```python
from build123d import *

# Parameters (mm, degrees)
SKETCH_1_W               = 100
SKETCH_1_H               = 228
EXTRUDE_1_DEPTH          = 1
SKETCH_2_W               = 96
SKETCH_2_H               = 1
SKETCH_2_W_2             = 1
SKETCH_2_H_2             = 224
EXTRUDE_2_DEPTH          = 23
FILLET_1_R               = 0.9
FILLET_2_R               = 1.9
CUT_EXTRUDE_1_DEPTH      = 22
CUT_EXTRUDE_1_DEPTH_BACK = 22
FILLET_3_R               = 1
SKETCH_4_R               = 5
CUT_EXTRUDE_2_DEPTH      = 10
SKETCH_5_R               = 2
CUT_EXTRUDE_3_DEPTH      = 30
SKETCH_6_R               = 2
CUT_EXTRUDE_4_DEPTH      = 30
SKETCH_7_R               = 2
CUT_EXTRUDE_5_DEPTH      = 30
SKETCH_8_R               = 2
CUT_EXTRUDE_6_DEPTH      = 30
CUT_EXTRUDE_7_DEPTH      = 10


with BuildPart() as part:
    # Эскиз1 → Бобышка-Вытянуть1 (new body)
    with BuildSketch(Plane.XY):
        with Locations((50, 114)):
            Rectangle(SKETCH_1_W, SKETCH_1_H)
    extrude(amount=EXTRUDE_1_DEPTH)

    # Эскиз2 → Бобышка-Вытянуть2 (add)
    with BuildSketch(Plane.XY.offset(1)):
        with Locations((50, 227.5)):
            Rectangle(SKETCH_2_W, SKETCH_2_H)
        with Locations((50, 0.5)):
            Rectangle(SKETCH_2_W, SKETCH_2_H)
        with Locations((99.5, 114)):
            Rectangle(SKETCH_2_W_2, SKETCH_2_H_2)
        with Locations((0.5, 114)):
            Rectangle(SKETCH_2_W_2, SKETCH_2_H_2)
    extrude(amount=EXTRUDE_2_DEPTH)

    # Скругление1
    fillet_1_edges = [part.edges().sort_by_distance(p)[0] for p in [
        (50, 227, 1),
        (50, 1, 1),
        (99, 114, 1),
        (1, 114, 1),
    ]]
    fillet(fillet_1_edges, radius=FILLET_1_R)

    # Скругление2
    # the kernel refuses this fillet: 1.9 mm, written as the material it takes off along each edge
    with BuildSketch(Plane(origin=(-4.75, 228, 0), x_dir=(0, -1, 0), z_dir=(1, 0, 0)), Plane(origin=(104.75, 0, 0), x_dir=(0, 1, 0), z_dir=(-1, 0, 0))) as fillet_2_piece_1:
        with BuildLine():
            CenterArc((FILLET_2_R, -FILLET_2_R), FILLET_2_R, 90, 90)
            Line((0, -FILLET_2_R), (0, 0))
            Line((0, 0), (FILLET_2_R, 0))
        make_face()
    extrude(amount=109.5, mode=Mode.SUBTRACT)
    with BuildSketch(Plane(origin=(100, 232.75, 0), x_dir=(-1, 0, 0), z_dir=(0, -1, 0))) as fillet_2_piece_2:
        with BuildLine():
            CenterArc((FILLET_2_R, -FILLET_2_R), FILLET_2_R, 90, 90)
            Line((0, -FILLET_2_R), (0, 0))
            Line((0, 0), (FILLET_2_R, 0))
        make_face()
    extrude(amount=237.5, mode=Mode.SUBTRACT)
    with BuildSketch(Plane(origin=(0, -4.75, 0), x_dir=(0, 0, 1), z_dir=(0, 1, 0))) as fillet_2_piece_3:
        with BuildLine():
            CenterArc((FILLET_2_R, FILLET_2_R), FILLET_2_R, 180, 90)
            Line((0, FILLET_2_R), (0, 0))
            Line((0, 0), (FILLET_2_R, 0))
        make_face()
    extrude(amount=237.5, mode=Mode.SUBTRACT)

    # Эскиз3 → Вырез-Вытянуть1 (cut, two sides: drawn at the far end of the back side and taken through both)
    with BuildSketch(Plane.XY.offset(1).offset(-CUT_EXTRUDE_1_DEPTH_BACK)):
        with BuildLine():
            Line((0.226679947, 226), (0.226679947, 227.773320053))
            Line((0.226679947, 227.773320053), (2, 227.773320053))
            Line((2, 227.773320053), (2, 226.329128785))
            ThreePointArc((2, 226.329128785), (2.076776695, 225.923223305), (1.670871215, 226))
            Line((1.670871215, 226), (0.226679947, 226))
        make_face()
        with BuildLine():
            Line((118, 226.329128785), (118, 227.773320053))
            Line((118, 227.773320053), (119.773320053, 227.773320053))
            Line((119.773320053, 227.773320053), (119.773320053, 226))
            Line((119.773320053, 226), (118.329128785, 226))
            ThreePointArc((118.329128785, 226), (117.923223305, 225.923223305), (118, 226.329128785))
        make_face()
        with BuildLine():
            Line((2, 1.670871215), (2, 0.226679947))
            Line((2, 0.226679947), (0.226679947, 0.226679947))
            Line((0.226679947, 0.226679947), (0.226679947, 2))
            Line((0.226679947, 2), (1.670871215, 2))
            ThreePointArc((1.670871215, 2), (2.076776695, 2.076776695), (2, 1.670871215))
        make_face()
        with BuildLine():
            Line((119.773320053, 2), (119.773320053, 0.226679947))
            Line((119.773320053, 0.226679947), (118, 0.226679947))
            Line((118, 0.226679947), (118, 1.670871215))
            ThreePointArc((118, 1.670871215), (117.923223305, 2.076776695), (118.329128785, 2))
            Line((118.329128785, 2), (119.773320053, 2))
        make_face()
    extrude(amount=CUT_EXTRUDE_1_DEPTH + CUT_EXTRUDE_1_DEPTH_BACK, mode=Mode.SUBTRACT)

    # Скругление3
    fillet_3_edges = [part.edges().sort_by_distance(p)[0] for p in [
        (98, 227.5, 24),
        (2, 227.5, 24),
        (98, 0.5, 24),
        (2, 0.5, 24),
        (99.5, 2, 24),
        (99.5, 226, 24),
        (0.5, 226, 24),
        (0.5, 2, 24),
    ]]
    fillet(fillet_3_edges, radius=FILLET_3_R)

    # Эскиз4 → Вырез-Вытянуть2 (cut)
    with BuildSketch(Plane.XY.offset(1)):
        with Locations((33.703708686, 202)):
            Circle(SKETCH_4_R)
        with Locations((33.703708686, 177)):
            Circle(SKETCH_4_R)
        with Locations((33.703708686, 152)):
            Circle(SKETCH_4_R)
        with Locations((33.703708686, 127)):
            Circle(SKETCH_4_R)
        with Locations((33.703708686, 102)):
            Circle(SKETCH_4_R)
        with Locations((33.703708686, 77)):
            Circle(SKETCH_4_R)
        with Locations((33.703708686, 52)):
            Circle(SKETCH_4_R)
        with Locations((33.703708686, 27)):
            Circle(SKETCH_4_R)
        with Locations((57.851854343, 20.529523872)):
            Circle(SKETCH_4_R)
        with Locations((57.851854343, 45.529523872)):
            Circle(SKETCH_4_R)
        with Locations((57.851854343, 70.529523872)):
            Circle(SKETCH_4_R)
        with Locations((57.851854343, 95.529523872)):
            Circle(SKETCH_4_R)
        with Locations((57.851854343, 120.529523872)):
            Circle(SKETCH_4_R)
        with Locations((57.851854343, 145.529523872)):
            Circle(SKETCH_4_R)
        with Locations((57.851854343, 170.529523872)):
            Circle(SKETCH_4_R)
        with Locations((57.851854343, 195.529523872)):
            Circle(SKETCH_4_R)
        with Locations((82, 202)):
            Circle(SKETCH_4_R)
        with Locations((82, 177)):
            Circle(SKETCH_4_R)
        with Locations((82, 152)):
            Circle(SKETCH_4_R)
        with Locations((82, 127)):
            Circle(SKETCH_4_R)
        with Locations((82, 102)):
            Circle(SKETCH_4_R)
        with Locations((82, 77)):
            Circle(SKETCH_4_R)
        with Locations((82, 52)):
            Circle(SKETCH_4_R)
        with Locations((82, 27)):
            Circle(SKETCH_4_R)
    extrude(amount=-CUT_EXTRUDE_2_DEPTH, mode=Mode.SUBTRACT)

    # Эскиз5 → Вырез-Вытянуть3 (cut)
    with BuildSketch(Plane(origin=(0, 228, 0), x_dir=(1, 0, 0), z_dir=(0, 1, 0))):
        with Locations(Location((16, -12, 0), (0, 0, 270))):
            Circle(SKETCH_5_R)
        with Locations(Location((84, -12, 0), (0, 0, 270))):
            Circle(SKETCH_5_R)
        with Locations((84, 252)):
            Circle(SKETCH_5_R)
        with Locations((16, 252)):
            Circle(SKETCH_5_R)
    extrude(amount=-CUT_EXTRUDE_3_DEPTH, mode=Mode.SUBTRACT)

    # Эскиз6 → Вырез-Вытянуть4 (cut)
    with BuildSketch(Plane(origin=(100, 0, 0), x_dir=(0, 0, -1), z_dir=(1, 0, 0))):
        with Locations((-12, 220)):
            Circle(SKETCH_6_R)
    extrude(amount=-CUT_EXTRUDE_4_DEPTH, mode=Mode.SUBTRACT)

    # Эскиз7 → Вырез-Вытянуть5 (cut)
    with BuildSketch(Plane(origin=(100, 0, 0), x_dir=(0, 0, -1), z_dir=(1, 0, 0))):
        with Locations((-12, 8)):
            Circle(SKETCH_7_R)
    extrude(amount=-CUT_EXTRUDE_5_DEPTH, mode=Mode.SUBTRACT)

    # Эскиз8 → Вырез-Вытянуть6 (cut)
    with BuildSketch(Plane.ZY):
        with Locations((12, 181.9)):
            Circle(SKETCH_8_R)
        with Locations((12, 46.3)):
            Circle(SKETCH_8_R)
        with Locations((12, 91.5)):
            Circle(SKETCH_8_R)
        with Locations((12, 136.7)):
            Circle(SKETCH_8_R)
    extrude(amount=-CUT_EXTRUDE_6_DEPTH, mode=Mode.SUBTRACT)

    # Эскиз9 → Вырез-Вытянуть7 (cut)
    with BuildSketch(Plane(origin=(0, 1, 0), x_dir=(1, 0, 0), z_dir=(0, 1, 0))):
        with BuildLine():
            Line((16, -9), (21, -9))
            ThreePointArc((21, -9), (26, -14), (21, -19))
            Line((21, -19), (16, -19))
            ThreePointArc((16, -19), (11, -14), (16, -9))
        make_face()
        with BuildLine():
            Line((84, -19), (79, -19))
            ThreePointArc((79, -19), (74, -14), (79, -9))
            Line((79, -9), (84, -9))
            ThreePointArc((84, -9), (89, -14), (84, -19))
        make_face()
    extrude(amount=-CUT_EXTRUDE_7_DEPTH, mode=Mode.SUBTRACT)


solid = part.part
```
CAD build for the part. Positions are in the model's coordinates, mm. A direction names the side the tool comes from. Give positions to 0.01 mm unless a question says otherwise; leave off trailing zeros. Order: outer loops, then holes, each group sorted by start corner. A loop starts at its lowest first (then second) coordinate and runs counter-clockwise, first axis right, second up.
(1) Mould opens along X. For faces 1 (the flat face through (100, 112, 13)), 2 (the flat face through (49, 1, 13)), 3 (the cylindrical face through (32.62, 72.12, 0.51)) say: released by +X, released by -X, zero draft, split by the parting line, or undercut.
(2) Saw through at B-B, the plane x = 8.5. Give the cut face in (y, z), then the cut area to 3 significant figures.
(3) Saw through at A-A, the plane z = 16.5. Give the cut face in (x, y).
(4) Drill centre lines: L1, parallel to X at y = 227.2, z = 12; L2, parallel to Y at x = 99.45, z = 12; L3, parallel to X at y = 79.5, z = 3.5. Where is each one in solid material? Low to high.
(5) Saw through at C-C, the plane x = 59.5. State how many separate pieces and enclosed holes the cut face has, then the cut area to 3 significant figures.
(6) Tool access for faces 4 (the cylindrical face through (26, 0.5, 13.9)), 5 (the flat face through (50, 116, 1)), 6 (the cylindrical face through (0.493, 48.283, 11.74)): list every direction of +Z, -Z, +X, -X, +Y, -Y with a clear straight run to the whole face (end or side of a thin tool).
(7) Flat gauge pins, fed straight in: pin 1 (1 mm diameter, centred on x = 99.5, z = 16, fed in from -Y); pin 2 (4.5 mm diameter, centred on y = 220, z = 12, fed in from -X); pin 3 (0.5 mm diameter, centred on y = 1, z = 12.5, fed in from -X); pin 4 (1.5 mm diameter, centred on y = 1, z = 7, fed in from +X). Where does each tip first touch, or does it go through?
Results found:
1. face 1: released by +X
1. face 2: zero draft
1. face 3: undercut
2. outline: (0, 1.9) arc R1.9 ccw to (1.9, 0) - (226.1, 0) arc R1.9 ccw to (228, 1.9) - (228, 24) - (227, 24) - (227, 1.9) arc R0.9 cw to (226.1, 1) - (1.9, 1) arc R0.9 cw to (1, 1.9) - (1, 24) - (0, 24) - close
2. area: 273 mm2
3. outline: (0, 2) - (1, 2) - (1, 226) - (0, 226) - close; (2, 0) - (11.67, 0) - (11.67, 1) - (2, 1) - close; (2, 227) - (98, 227) - (98, 228) - (2, 228) - close; (25.33, 0) - (74.67, 0) - (74.67, 1) - (25.33, 1) - close; (88.33, 0) - (98, 0) - (98, 1) - (88.33, 1) - close; (99, 2) - (100, 2) - (100, 226) - (99, 226) - close
4. L1: x = 2 to 14, 18 to 82, 86 to 98
4. L2: y = 2 to 6, 10 to 218, 222 to 226
4. L3: x = 0 to 1, 99 to 100
5. separate pieces: 9
5. enclosed holes: 0
5. area: 197 mm2
6. face 4: -Y
6. face 5: +Z
6. face 6: -X
7. pin 1: stops at y = 2
7. pin 2: stops at x = 0
7. pin 3: stops at x = 2
7. pin 4: stops at x = 98
